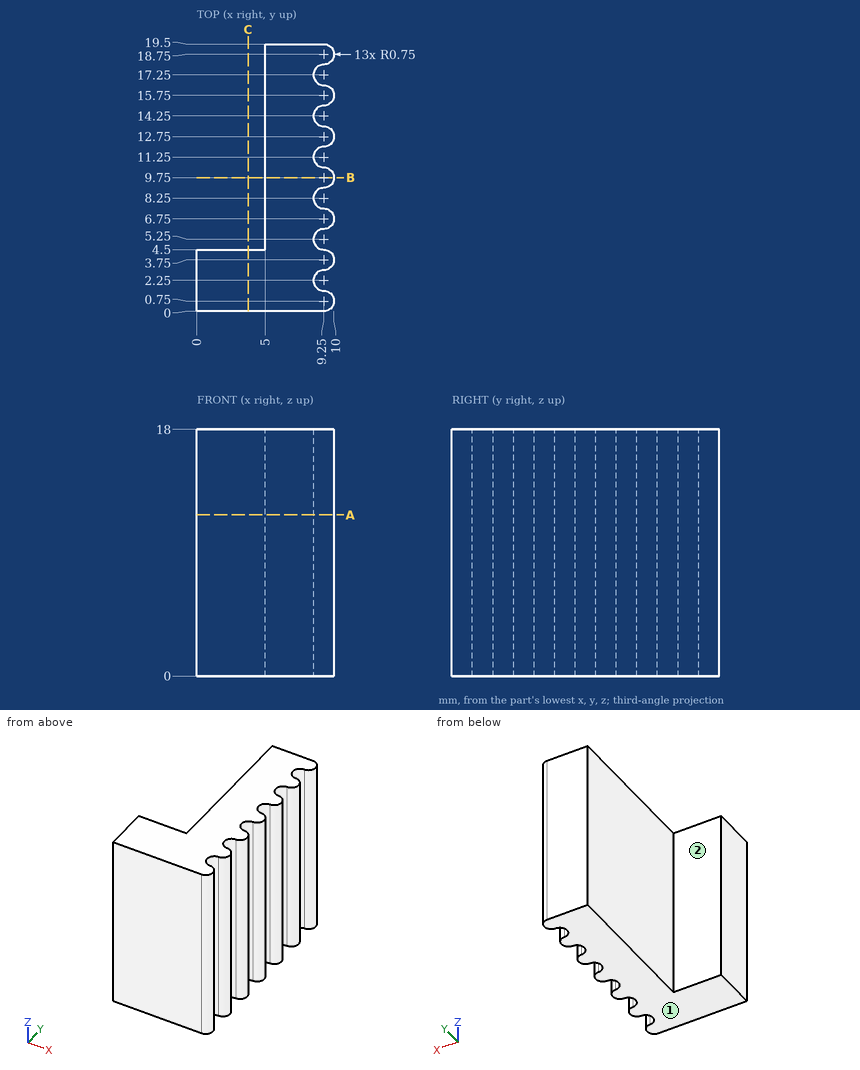
Verification items for this drawing (mm, ordinates from the low corner). A direction names the side the tool comes from. Round coordinates to 2 decimals unless told otherwise and drop trailing zeros. Loops run counter-clockwise (first coordinate to the right, second up) from the corner with the lowest first, then second, coordinate; pieces in that order, holes last. Notation, with made-up numbers: (82, -13.5) - (87, -13.5) arc R10 ccw to (87, 3.5) - close; hole circle Ø11 at (-10, -29). An arc over 180 degrees is marked (long way). Answer as CSV lines item,"result". Start each with the question number.
Item 1: Set-up check for the marked faces 1 and 2: record each of +Z, -Z, +X, -X, +Y, -Y from which the full face is reachable in a straight line by a thin tool's end or side.
Item 2: Scan lines: line 1 (X direction, y = 5.25, z = 6.5); line 2 (X direction, y = 6.75, z = 1); line 3 (Y direction, x = 1, z = 4.5). Record each from-to range of solid material in increasing order. Write a range as [from, to].
Item 3: Section check A-A (z = 11.75). Record the boundary of the cut face in (x, y).
Item 4: Section check B-B (y = 9.75). Record the boundary of the cut face in (x, z), and give its area (3 significant figures).
Item 5: Section check C-C (x = 3.75). Record the boundary of the cut face in (y, z), and give its area (3 significant figures).
Item 6: Depth check by flat-ended pin: P1, Ø3, axis at y = 13, z = 11.5, coming from the -X side; P2, Ø4, axis at x = 2, z = 9, coming from the +Y side. Enter the tip coordinate at first touch or a pass-through.
Report:
1,face 1,"-Z, +X, -X, +Y, -Y"
1,face 2,"+Z, -Z, -X, +Y"
2,line 1,"x = [5, 8.5]"
2,line 2,"x = [5, 10]"
2,line 3,"y = [0, 4.5]"
3,outline,"(0, 0) - (9.25, 0) arc R0.75 ccw to (9.25, 1.5) arc R0.75 cw to (9.25, 3) arc R0.75 ccw to (9.25, 4.5) arc R0.75 cw to (9.25, 6) arc R0.75 ccw to (9.25, 7.5) arc R0.75 cw to (9.25, 9) arc R0.75 ccw to (9.25, 10.5) arc R0.75 cw to (9.25, 12) arc R0.75 ccw to (9.25, 13.5) arc R0.75 cw to (9.25, 15) arc R0.75 ccw to (9.25, 16.5) arc R0.75 cw to (9.25, 18) arc R0.75 ccw to (9.25, 19.5) - (5, 19.5) - (5, 4.5) - (0, 4.5) - close"
4,outline,"(5, 0) - (10, 0) - (10, 18) - (5, 18) - close"
4,area,"90.0 mm2"
5,outline,"(0, 0) - (4.5, 0) - (4.5, 18) - (0, 18) - close"
5,area,"81.0 mm2"
6,P1,"stops at x = 5"
6,P2,"stops at y = 4.5"
